For this review, take the finished solid that the model builds, in its own axes (mm). Face numbers are marked on the shaded views. A direction names the side the tool comes from. Coordinates: 2 decimals unless noted, no trailing zeros. Write each loop counter-clockwise with the first axis right and the second up, starting at its lowest first coordinate (ties: lowest second). Pieces come first, ordered by that corner, then holes. Notation, with made-up numbers: M -27.5,85.25 L -8.5,85.25 A21 ccw -8.5,111.25 Z; hole C -34.75,25.5 d6. An arc over 180 degrees is marked long. One line per question, with ' | ' between items.
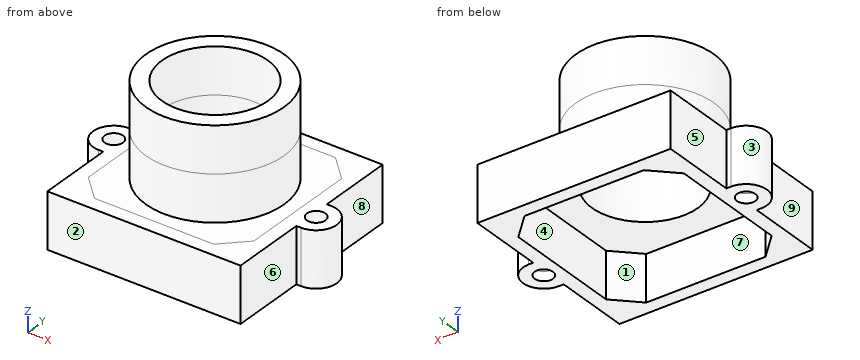
from build123d import *
from build123d.topology import SkipClean

# Parameters (mm, degrees)
BASE_HULL_DEPTH                   = 5
BASE_START                        = 1
BASE_COVER_DEPTH                  = 1
LENS_HOLE_HULL_BASE_SKETCH_R      = 7.5
LENS_HOLE_HULL_DEPTH              = 10
LENS_HOLE_D                       = 11.5
MOUNT_HOLES_D                     = 2
PULL_START                        = -5
PULL_BASE_TO_ORIGIN_OUTLINE_R     = 1
PULL_BASE_TO_ORIGIN_DEPTH         = 5
PULL_BASE_TO_ORIGIN_2_OUTLINE_R   = 5.75
PULL_BASE_TO_ORIGIN_2_DEPTH       = 5
PULL_START_2                      = 1
PULL_BASE_TO_ORIGIN_3_OUTLINE_R   = 1
PULL_BASE_TO_ORIGIN_3_DEPTH       = 5
PULL_START_3                      = 11
PULL_BASE_TO_ORIGIN_4_OUTLINE_R   = 7.5
PULL_BASE_TO_ORIGIN_4_OUTLINE_R_2 = 5.75
PULL_BASE_TO_ORIGIN_4_DEPTH       = 5
PULL_START_4                      = 5
PULL_BASE_TO_ORIGIN_5_OUTLINE_R   = 7.5
PULL_BASE_TO_ORIGIN_5_DEPTH       = 1


# Read off the part's stored shape, not the designer's step: Pull base to origin
with BuildPart() as part:
    # Base sketch → Base hull (new body)
    with BuildSketch(Plane.XY):
        with BuildLine():
            Line((-10.5, 10.5), (10.5, 10.5))
            Line((10.5, 10.5), (10.5, 2.25))
            Line((10.5, 2.25), (11, 2.25))
            ThreePointArc((11, 2.25), (13.25, 0), (11, -2.25))
            Line((11, -2.25), (10.5, -2.25))
            Line((10.5, -2.25), (10.5, -10.5))
            Line((10.5, -10.5), (-10.5, -10.5))
            Line((-10.5, -10.5), (-10.5, -2.25))
            Line((-10.5, -2.25), (-11, -2.25))
            ThreePointArc((-11, -2.25), (-13.25, 0), (-11, 2.25))
            Line((-11, 2.25), (-10.5, 2.25))
            Line((-10.5, 2.25), (-10.5, 10.5))
        make_face()
        Polygon((-9, 6.485638508), (-9, -6.485638508), (-6.485638508, -9), (6.485638508, -9), (9, -6.485638508), (9, 6.485638508), (6.485638508, 9), (-6.485638508, 9), align=None, mode=Mode.SUBTRACT)
    extrude(amount=-BASE_HULL_DEPTH)

    # Base sketch<2> → Base cover (add)
    # profile 1 of 2: a face of its own
    with BuildSketch(Plane.XY.offset(BASE_START)):
        with BuildLine():
            ThreePointArc((11, 2.25), (13.25, 0), (11, -2.25))
            Line((11, -2.25), (10.5, -2.25))
            Line((10.5, -2.25), (10.5, -10.5))
            Line((10.5, -10.5), (-10.5, -10.5))
            Line((-10.5, -10.5), (-10.5, -2.25))
            Line((-10.5, -2.25), (-11, -2.25))
            ThreePointArc((-11, -2.25), (-13.25, 0), (-11, 2.25))
            Line((-11, 2.25), (-10.5, 2.25))
            Line((-10.5, 2.25), (-10.5, 10.5))
            Line((-10.5, 10.5), (10.5, 10.5))
            Line((10.5, 10.5), (10.5, 2.25))
            Line((10.5, 2.25), (11, 2.25))
        make_face()
        Polygon((-6.485638508, 9), (-9, 6.485638508), (-9, -6.485638508), (-6.485638508, -9), (6.485638508, -9), (9, -6.485638508), (9, 6.485638508), (6.485638508, 9), align=None, mode=Mode.SUBTRACT)
    # profile 2 of 2: a face of its own
    with BuildSketch(Plane.XY.offset(BASE_START)):
        Polygon((6.485638508, 9), (-6.485638508, 9), (-9, 6.485638508), (-9, -6.485638508), (-6.485638508, -9), (6.485638508, -9), (9, -6.485638508), (9, 6.485638508), align=None)
    extrude(amount=-BASE_COVER_DEPTH)

    # Lens hole hull base sketch → Lens hole hull (add)
    with BuildSketch(Plane.XY.offset(1)):
        Circle(LENS_HOLE_HULL_BASE_SKETCH_R)
    extrude(amount=LENS_HOLE_HULL_DEPTH)

    # Lens hole (through all)
    with Locations(Plane.XY.offset(11)):
        with Locations((0, 0)):
            Hole(LENS_HOLE_D / 2)

    # Mount holes (through all)
    with Locations(Plane.XY.offset(1)):
        with Locations((-11, 0), (11, 0)):
            Hole(MOUNT_HOLES_D / 2)

    # Pull base to origin outline → Pull base to origin (cut)
    with BuildSketch(Plane.XY.offset(PULL_START)):
        with BuildLine():
            Line((10.5, 10.5), (-10.5, 10.5))
            Line((-10.5, 10.5), (-10.5, 2.25))
            Line((-10.5, 2.25), (-11, 2.25))
            ThreePointArc((-11, 2.25), (-13.25, 0), (-11, -2.25))
            Line((-11, -2.25), (-10.5, -2.25))
            Line((-10.5, -2.25), (-10.5, -10.5))
            Line((-10.5, -10.5), (10.5, -10.5))
            Line((10.5, -10.5), (10.5, -2.25))
            Line((10.5, -2.25), (11, -2.25))
            ThreePointArc((11, -2.25), (13.25, 0), (11, 2.25))
            Line((11, 2.25), (10.5, 2.25))
            Line((10.5, 2.25), (10.5, 10.5))
        make_face()
        with Locations((-11, 0)):
            Circle(PULL_BASE_TO_ORIGIN_OUTLINE_R, mode=Mode.SUBTRACT)
        Polygon((6.485638508, -9), (-6.485638508, -9), (-9, -6.485638508), (-9, 6.485638508), (-6.485638508, 9), (6.485638508, 9), (9, 6.485638508), (9, -6.485638508), align=None, mode=Mode.SUBTRACT)
        with Locations((11, 0)):
            Circle(PULL_BASE_TO_ORIGIN_OUTLINE_R, mode=Mode.SUBTRACT)
    extrude(amount=PULL_BASE_TO_ORIGIN_DEPTH, mode=Mode.SUBTRACT)

    # Pull base to origin 2 outline → Pull base to origin 2 (cut)
    with BuildSketch(Plane.XY):
        Polygon((-9, -6.485638508), (-6.485638508, -9), (6.485638508, -9), (9, -6.485638508), (9, 6.485638508), (6.485638508, 9), (-6.485638508, 9), (-9, 6.485638508), align=None)
        Circle(PULL_BASE_TO_ORIGIN_2_OUTLINE_R, mode=Mode.SUBTRACT)
    extrude(amount=PULL_BASE_TO_ORIGIN_2_DEPTH, mode=Mode.SUBTRACT)

    # Pull base to origin 3 outline → Pull base to origin 3 (add)
    with SkipClean():  # the faces are left unmerged after this step: merging them gives an invalid solid
        with BuildSketch(Plane.XY.offset(PULL_START_2)):
            with BuildLine():
                Line((10.5, 10.5), (-10.5, 10.5))
                Line((-10.5, 10.5), (-10.5, 2.25))
                Line((-10.5, 2.25), (-11, 2.25))
                ThreePointArc((-11, 2.25), (-13.25, 0), (-11, -2.25))
                Line((-11, -2.25), (-10.5, -2.25))
                Line((-10.5, -2.25), (-10.5, -10.5))
                Line((-10.5, -10.5), (10.5, -10.5))
                Line((10.5, -10.5), (10.5, -2.25))
                Line((10.5, -2.25), (11, -2.25))
                ThreePointArc((11, -2.25), (13.25, 0), (11, 2.25))
                Line((11, 2.25), (10.5, 2.25))
                Line((10.5, 2.25), (10.5, 10.5))
            make_face()
            with Locations((-11, 0)):
                Circle(PULL_BASE_TO_ORIGIN_3_OUTLINE_R, mode=Mode.SUBTRACT)
            Polygon((6.485638508, -9), (-6.485638508, -9), (-9, -6.485638508), (-9, 6.485638508), (-6.485638508, 9), (6.485638508, 9), (9, 6.485638508), (9, -6.485638508), align=None, mode=Mode.SUBTRACT)
            with Locations((11, 0)):
                Circle(PULL_BASE_TO_ORIGIN_3_OUTLINE_R, mode=Mode.SUBTRACT)
        extrude(amount=PULL_BASE_TO_ORIGIN_3_DEPTH)
    add(part.part.scale(1), mode=Mode.REPLACE)  # the faces are merged on a copy

    # Pull base to origin 4 outline → Pull base to origin 4 (add)
    with SkipClean():  # the faces are left unmerged after this step: merging them gives an invalid solid
        with BuildSketch(Plane.XY.offset(PULL_START_3)):
            Circle(PULL_BASE_TO_ORIGIN_4_OUTLINE_R)
            Circle(PULL_BASE_TO_ORIGIN_4_OUTLINE_R_2, mode=Mode.SUBTRACT)
        extrude(amount=PULL_BASE_TO_ORIGIN_4_DEPTH)

    # Pull base to origin 5 outline → Pull base to origin 5 (add)
    with SkipClean():  # the faces are left unmerged after this step: merging them gives an invalid solid
        with BuildSketch(Plane.XY.offset(PULL_START_4)):
            Polygon((-9, -6.485638508), (-6.485638508, -9), (6.485638508, -9), (9, -6.485638508), (9, 6.485638508), (6.485638508, 9), (-6.485638508, 9), (-9, 6.485638508), align=None)
            Circle(PULL_BASE_TO_ORIGIN_5_OUTLINE_R, mode=Mode.SUBTRACT)
        extrude(amount=PULL_BASE_TO_ORIGIN_5_DEPTH)


solid = part.part
1. Take a section at C-C on y = -4.5. State the section outline as (x, z) points.
Computed values:
outline: M -10.5,0 L -9,0 L -9,5 L -3.58,5 L -3.58,16 L -6,16 L -6,6 L -10.5,6 Z; M 3.58,5 L 9,5 L 9,0 L 10.5,0 L 10.5,6 L 6,6 L 6,16 L 3.58,16 Z
2. Clearance check with flat-ended pins moving along their axes: P1, Ø2.5, axis at x = 11, y = 0, coming from the -Z side; P2, Ø6.5, axis at y = -8.5, z = 3, coming from the +X side; P3, Ø1.6, axis at x = -11, y = 0, coming from the +Z side; P4, Ø5, axis at y = -8, z = 3, coming from the -X side. State where each tip first meets the part, or that it passes through.
Computed values:
P1: stops at z = 0 | P2: stops at x = 10.5 | P3: passes through | P4: stops at x = -10.5
3. Take a section at A-A on y = 0. State the section outline as (x, z) points, plus the area to 3 significant figures.
Computed values:
outline: M -13.25,0 L -12,0 L -12,6 L -13.25,6 Z; M -10,0 L -9,0 L -9,5 L -5.75,5 L -5.75,16 L -7.5,16 L -7.5,6 L -10,6 Z; M 5.75,5 L 9,5 L 9,0 L 10,0 L 10,6 L 7.5,6 L 7.5,16 L 5.75,16 Z; M 12,0 L 13.25,0 L 13.25,6 L 12,6 Z | area: 68.5 mm2
4. Machinability: for the marked faces 5, 6, 7, 8 and 9, which of the approach directions +Z, -Z, +X, -X, +Y, -Y give a long, thin tool a straight path to every point of the face, cutting with its end or side? Answer none if there is none.
Computed values:
face 5: +Z, -Z, -X, +Y | face 6: +Z, -Z, +X, -Y | face 7: -Z | face 8: +Z, -Z, +X, +Y | face 9: +Z, -Z, -X, -Y
5. For line 1 along X through (y, z) = (-2.75, 2.25); line 2 along Y through (x, z) = (11, 0.8), list the stretches that pass through material, from the lowest coordinate up.
Computed values:
line 1: x = -10.5 to -9, 9 to 10.5 | line 2: y = -2.25 to -1, 1 to 2.25
6. Take a section at D-D on z = 13. State the section outline as (x, y) points.
Computed values:
outline: C 0,0 d15; hole C 0,0 d11.5
7. Take a section at B-B on x = 4. State the section outline as (y, z) points, plus the area to 3 significant figures.
Computed values:
outline: M -10.5,0 L -9,0 L -9,5 L -4.13,5 L -4.13,16 L -6.34,16 L -6.34,6 L -10.5,6 Z; M 4.13,5 L 9,5 L 9,0 L 10.5,0 L 10.5,6 L 6.34,6 L 6.34,16 L 4.13,16 Z | area: 72.0 mm2
8. Draft analysis for pull direction X (two halves, no side actions). For the marked faces 1, 2, 3 and 4, state which applies: pulls with the +X half, pulls with the -X half, needs draft (parallel to the pull), parting line crosses it, or undercut.
Computed values:
face 1: undercut | face 2: needs draft | face 3: pulls with the -X half | face 4: undercut
